from build123d import *

# Parameters (mm, degrees)
F0_W     = 280
F0_H     = 30
F1_DEPTH = 3
F2_W     = 20
F2_H     = 3
F3_DEPTH = 3
F4_W     = 3
F4_H     = 7.5
F5_DEPTH = 25


with BuildPart() as f1:
    # F0 (on Right) → F1 (new body)
    with BuildSketch(Plane.YZ):
        Rectangle(F0_W, F0_H)
    extrude(amount=F1_DEPTH)

    # F2 (on face) → F3 (join, through all)
    with BuildSketch(Plane.YZ.offset(3)):
        with Locations((120, -16.5)):
            Rectangle(F2_W, F2_H)
        with Locations((80, -16.5)):
            Rectangle(F2_W, F2_H)
        with Locations((40, -16.5)):
            Rectangle(F2_W, F2_H)
        with Locations((0, -16.5)):
            Rectangle(F2_W, F2_H)
        with Locations((-40, -16.5)):
            Rectangle(F2_W, F2_H)
        with Locations((-80, -16.5)):
            Rectangle(F2_W, F2_H)
        with Locations((-120, -16.5)):
            Rectangle(F2_W, F2_H)
    extrude(amount=-F3_DEPTH)

    # F4 (on face) → F5 (cut)
    with BuildSketch(Plane.YZ.offset(3)):
        with Locations((120, -3.75)):
            Rectangle(F4_W, F4_H)
        with Locations((80, -3.75)):
            Rectangle(F4_W, F4_H)
        with Locations((40, -3.75)):
            Rectangle(F4_W, F4_H)
        with Locations((0, -3.75)):
            Rectangle(F4_W, F4_H)
        with Locations((-40, -3.75)):
            Rectangle(F4_W, F4_H)
        with Locations((-80, -3.75)):
            Rectangle(F4_W, F4_H)
        with Locations((-120, -3.75)):
            Rectangle(F4_W, F4_H)
    extrude(amount=-F5_DEPTH, mode=Mode.SUBTRACT)


solid = f1.part
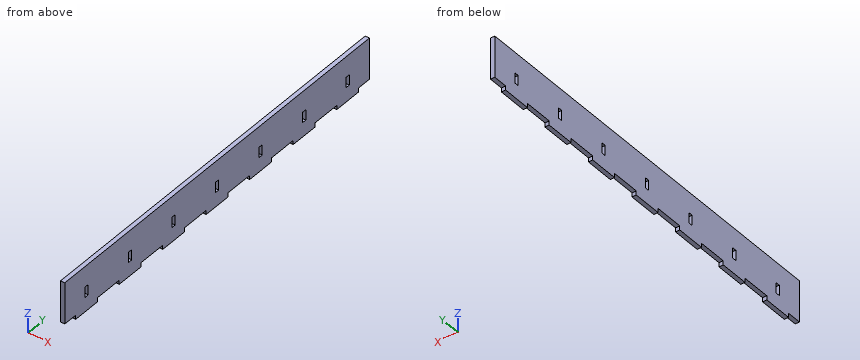
Could you check a few things on this model? Use its own coordinates, in mm. Coordinates: 2 decimals unless noted, no trailing zeros. Loops run counter-clockwise (first coordinate to the right, second up) from the corner with the lowest first, then second, coordinate; pieces in that order, holes last.
1. I need wall thicknesses on L1, parallel to Z at x = 1.15, y = 103.5; L2, parallel to Z at x = 0.25, y = 39. Which ranges of each line are inside material? Lowest first, please.
2. Imagine slicing it at B-B (x = 0.5). Give the number of separate pieces and of enclosed holes in the cut face, and give its area (3 significant figures).
3. For P1, Ø1.5, axis at y = -55, z = -13.5, coming from the -X side; P2, Ø0.9, axis at x = 2, y = 136.5, coming from the -Z side; P3, Ø0.9, axis at x = 1.5, z = -16, coming from the +Y side; P4, Ø0.9, axis at x = 2, z = -17, coming from the -Y side, each with a flat end and sliding along its axis, tell me the tip position at first contact or that it passes through.
4. Imagine slicing it at A-A (y = -105). Please give me the cut outline in (x, z), and give its area (3 significant figures).
Computed values:
1. L1: z = -15 to 15
1. L2: z = -18 to -7.5, 0 to 15
2. separate pieces: 1
2. enclosed holes: 7
2. area: 8,660 mm2
3. P1: stops at x = 0
3. P2: stops at z = -15
3. P3: stops at y = 130
3. P4: stops at y = -130
4. outline: (0, -15) - (3, -15) - (3, 15) - (0, 15) - close
4. area: 90.0 mm2
